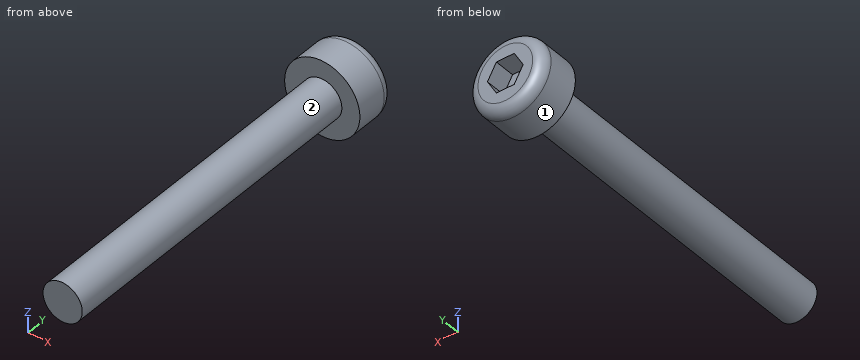
Autodesk Inventor part; units mm, degrees
ref_plane "YZ Plane" through (0, 0, 0) normal (1, 0, 0) x (0, 1, 0)
ref_plane "XZ Plane" through (0, 0, 0) normal (0, 1, 0) x (-1, 0, 0)
ref_plane "XY Plane" through (0, 0, 0) normal (0, 0, 1) x (1, 0, 0)
sketch "Sketch1" plane through (0, 0, 0) normal (0, 1, 0) x (-1, 0, 0)
  circle A0 centre (0, 0) radius 0.95
  circle A1 centre (0, 0) radius 1.825
  line L0 (0.433, -0.75) -> (-0.433, -0.75)
  line L1 (-0.433, -0.75) -> (-0.866, 0)
  line L2 (-0.866, 0) -> (-0.433, 0.75)
  line L3 (-0.433, 0.75) -> (0.433, 0.75)
  line L4 (0.433, 0.75) -> (0.866, 0)
  line L5 (0.866, 0) -> (0.433, -0.75)
  dimension "d0" = 1.9
  dimension "d1" = 3.65
  dimension "d8" = 1.5
extrude "Extrusion1" add sketch "Sketch1" along normal blind 2 contours A0 | A1 | L0 L1 L2 L3 L4 L5
extrude "Extrusion2" add sketch "Sketch1" against normal blind 16 contours A0 | L0 L1 L2 L3 L4 L5
extrude "Extrusion3" cut sketch "Sketch1" against normal blind 1 from surface at 2 contours L0 L1 L2 L3 L4 L5
fillet "Fillet1" radius 0.5 1 edges at (1.825, 2, 0)
thread "Thread2"
equation "\"d4\" = length"
equation "\"length\" = 16"
properties part number "M2x16"
The model under review builds one solid part; all positions refer to its coordinate system, in mm. Face numbers are marked on the shaded views. A direction names the side the tool comes from. Coordinates: 2 decimals unless noted, no trailing zeros. Write each loop counter-clockwise with the first axis right and the second up, starting at its lowest first coordinate (ties: lowest second). Pieces come first, ordered by that corner, then holes.
1) Machinability: for the marked faces 1 and 2, which of the approach directions +Z, -Z, +X, -X, +Y, -Y give a long, thin tool a straight path to every point of the face, cutting with its end or side? Answer none if there is none.
2) To check wall thickness, follow probe 1 along Y at (x, z) = (-1.3, -0.2); probe 2 along X at (y, z) = (-1.25, -0.5); probe 3 along X at (y, z) = (-14, -0.85). State the ranges of each line that lie inside material, in increasing order.
3) We need section A-A on x = 0. State the section outline as (y, z) points (3 decimals), then the cut area to 3 significant figures.
4) Clearance check with a flat-ended pin moving along its axis: pin 1 Ø0.8 at (x, z) = (0, -0.5) entering from +Y. State where the tip first meets the part, or that it passes through.
5) We need section B-B on y = -6. State the section outline as (x, z) points, then the cut area to 3 significant figures.
Answer list:
1. face 1: +Y, -Y
1. face 2: -Y
2. probe 1: y = 0 to 2
2. probe 2: x = -0.81 to 0.81
2. probe 3: x = -0.42 to 0.42
3. outline: (-16, -0.95) - (0, -0.95) - (0, -1.825) - (1.5, -1.825) arc R0.5 ccw to (2, -1.325) - (2, -0.75) - (1, -0.75) - (1, 0.75) - (2, 0.75) - (2, 1.325) arc R0.5 ccw to (1.5, 1.825) - (0, 1.825) - (0, 0.95) - (-16, 0.95) - close
3. area: 36.1 mm2
4. pin 1: stops at y = 2
5. outline: circle Ø1.9 at (0, 0)
5. area: 2.84 mm2
